Model file for the job. Use its own axes, mm. A direction names the side the tool comes from. Round coordinates to 2 decimals unless told otherwise and drop trailing zeros. Order: outer loops, then holes, each group sorted by start corner. A loop starts at its lowest first (then second) coordinate and runs counter-clockwise, first axis right, second up. Notation, with made-up numbers: (-22.5, 14.5) - (3.5, 14.5) arc R35 ccw to (3.5, 48.5) - close; hole circle Ø8 at (46.5, 8.5). An arc over 180 degrees is marked (long way). Write item = value, one per line.
```python
from build123d import *

# Parameters (mm, degrees)
F1_DEPTH = 30
F2_R     = 1.1
F3_DEPTH = 32.301
F4_W     = 29.3
F4_H     = 1.5
F5_DEPTH = 40
F6_W     = 5.2225396744
F6_H     = 13
F7_DEPTH = 32.301
F8_R     = 1
F8_R_2   = 4
F9_DEPTH = 1.5
F10_R    = 1


with BuildPart() as f1:
    # F0 (on Front) → F1 (new body)
    with BuildSketch(Plane.XZ):
        Polygon((0, 41.5), (0, 0), (1.5, 0), (1.5, 40), (30.8, 40), (30.8, 0), (32.3, 0), (32.3, 41.5), align=None)
    extrude(amount=F1_DEPTH)

    # F2 (on face) → F3 (cut, through all)
    with BuildSketch(Plane(origin=(0, 0, 0), x_dir=(0, -1, 0), z_dir=(-1, 0, 0))):
        with BuildLine():
            Line((19, 0), (19, 15))
            ThreePointArc((19, 15), (15, 19), (11, 15))
            Line((11, 15), (11, 0))
            Line((11, 0), (19, 0))
        make_face()
        with Locations((21.2225396744, 15)):
            Circle(F2_R)
        with Locations((19.4, 19.4)):
            Circle(F2_R)
        with Locations((15, 21.2225396744)):
            Circle(F2_R)
        with Locations((10.6, 19.4)):
            Circle(F2_R)
        with Locations((8.7774603256, 15)):
            Circle(F2_R)
    extrude(amount=-F3_DEPTH, mode=Mode.SUBTRACT)

    # F4 (on face) → F5 (join)
    with BuildSketch(Plane(origin=(0, 0, 40), x_dir=(1, 0, 0), z_dir=(0, 0, -1))):
        with Locations((16.15, 29.25)):
            Rectangle(F4_W, F4_H)
    extrude(amount=F5_DEPTH)

    # F6 (on face) → F7 (cut, through all)
    with BuildSketch(Plane(origin=(0, 0, 0), x_dir=(0, -1, 0), z_dir=(-1, 0, 0))):
        Polygon((30, 41.5), (0, 41.5), (0, 26.5), (0, 0), (5.7774603256, 0), (5.7774603256, 13), (5.7774603256, 26.5), (30, 26.5), align=None)
        with Locations((8.3887301628, 6.5)):
            Rectangle(F6_W, F6_H)
        Polygon((28.5, 1.7727272727), (19, 13), (19, 0), (30, 0), align=None)
        Polygon((30, 0), (30, 1.7727272727), (28.5, 1.7727272727), align=None)
    extrude(amount=-F7_DEPTH, mode=Mode.SUBTRACT)

    # F8 (on face) → F9 (cut, through all)
    with BuildSketch(Plane.XZ.offset(30)):
        with Locations((6.15, 24.1363636364)):
            Circle(F8_R)
        with Locations((6.15, 4.1363636364)):
            Circle(F8_R)
        with Locations((26.15, 24.1363636364)):
            Circle(F8_R)
        with Locations((26.15, 4.1363636364)):
            Circle(F8_R)
        with Locations((16.15, 14.1363636364)):
            Circle(F8_R_2)
        with Locations((20.55, 18.5363636364)):
            Circle(F8_R)
        with Locations((16.15, 20.3589033108)):
            Circle(F8_R)
        with Locations((11.75, 18.5363636364)):
            Circle(F8_R)
        with Locations((9.9274603256, 14.1363636364)):
            Circle(F8_R)
        with Locations((11.75, 9.7363636364)):
            Circle(F8_R)
        with Locations((16.15, 7.9138239619)):
            Circle(F8_R)
        with Locations((20.55, 9.7363636364)):
            Circle(F8_R)
        with Locations((22.3725396744, 14.1363636364)):
            Circle(F8_R)
    extrude(amount=-F9_DEPTH, mode=Mode.SUBTRACT)

    # F10
    f10_edges = [f1.edges().sort_by_distance(p)[0] for p in [
        (0.75, -5.77746, 13),
        (31.55, -5.77746, 13),
        (0.75, -19, 13),
        (31.55, -19, 13),
        (0.75, -11, 13),
        (31.55, -11, 13),
        (31.55, -5.77746, 26.5),
        (0.75, -5.77746, 26.5),
    ]]
    fillet(f10_edges, radius=F10_R)


solid = f1.part
```
1) Cut at B-B (x = 26.15). Write the cut outline in (y, z).
Conclusion:
outline = (-30, 1.77) - (-28.5, 1.77) - (-28.5, 3.14) - (-30, 3.14) - close; (-30, 5.14) - (-28.5, 5.14) - (-28.5, 23.14) - (-30, 23.14) - close; (-30, 25.14) - (-28.5, 25.14) - (-28.5, 26.5) - (-30, 26.5) - close
2) 3-axis set-ups, long thin cutter, end or side, ignore diameter. For faces 1 (the face through (0.7, -11, 14.5)), 2 (the face through (1, -8, 13)), 3 (the face through (11, -29.3, 10.4)): which of +Z, -Z, +X, -X, +Y, -Y reach the whole face in a straight line?
Conclusion:
face_1 = -Z, +X, -X
face_2 = -Z, +X, -X, +Y
face_3 = +Y, -Y
3) Cut at C-C (z = 11.75). Write the cut outline in (x, y), and give its area (3 significant figures).
Conclusion:
outline = (0, -30) - (12.94, -30) - (12.94, -28.5) - (1.5, -28.5) - (1.5, -20.06) - (0, -20.06) - close; (19.36, -30) - (32.3, -30) - (32.3, -20.06) - (30.8, -20.06) - (30.8, -28.5) - (19.36, -28.5) - close
area = 64.1 mm^2
4) Wall check: line 1 along Z through (x, y) = (16.15, -28.9); line 2 along X through (y, z) = (-23, 25.5); line 3 along Z through (x, y) = (12, -29). Give the ranges that are in metal, low to high.
Conclusion:
line_1 = 1.77 to 6.91, 8.91 to 10.14, 18.14 to 19.36, 21.36 to 26.5
line_2 = 0 to 1.5, 30.8 to 32.3
line_3 = 1.77 to 8.77, 10.7 to 17.57, 19.5 to 26.5
5) Cut at D-D (x = 16.15). Write the cut outline in (y, z), and give its area (3 significant figures).
Conclusion:
outline = (-30, 1.77) - (-28.5, 1.77) - (-28.5, 6.91) - (-30, 6.91) - close; (-30, 8.91) - (-28.5, 8.91) - (-28.5, 10.14) - (-30, 10.14) - close; (-30, 18.14) - (-28.5, 18.14) - (-28.5, 19.36) - (-30, 19.36) - close; (-30, 21.36) - (-28.5, 21.36) - (-28.5, 26.5) - (-30, 26.5) - close
area = 19.1 mm^2
6) Flat gauge pins, fed straight in: pin 1 Ø3 at (x, z) = (22.37, 14.14) entering from +Y; pin 2 Ø2 at (y, z) = (-14.5, 22.5) entering from -X; pin 3 Ø1.6 at (x, y) = (0.5, -8) entering from -Z. Where does each tip first touch, or does it go through?
Conclusion:
pin_1 = -28.5
pin_2 = 0
pin_3 = 13
7) Cut at A-A (y = -10.6). Write the cut outline in (x, z), and give its area (3 significant figures).
Conclusion:
outline = (0, 13.2) - (1.5, 13.2) - (1.5, 18.3) - (0, 18.3) - close; (0, 20.5) - (1.5, 20.5) - (1.5, 26.5) - (0, 26.5) - close; (30.8, 13.2) - (32.3, 13.2) - (32.3, 18.3) - (30.8, 18.3) - close; (30.8, 20.5) - (32.3, 20.5) - (32.3, 26.5) - (30.8, 26.5) - close
area = 33.3 mm^2
8) Mould opens along X. For faces 4 (the face through (16, -29, 1.773)), 5 (the face through (16.02, -29.26, 8.905)), 6 (the face through (32.3, -20, 17)) say: +X half, -X half, draft (parallel to the pull), parting line (faces both ways), or undercut.
Conclusion:
face_4 = draft
face_5 = undercut
face_6 = +X half
